Check sheet for the modelled part. Datum: model origin and axes. Units: mm. A direction names the side the tool comes from. Coordinates: 2 decimals unless noted, no trailing zeros. Loops run counter-clockwise (first coordinate to the right, second up) from the corner with the lowest first, then second, coordinate; pieces in that order, holes last. Notation, with made-up numbers: (10, 45.25) -> (23, 45.25) arc R28 ccw to (23, 76.25) -> close; hole circle Ø1 at (50.25, 72). An arc over 180 degrees is marked (long way). Use one line per item in the form item = value.
from build123d import *

# Parameters (mm, degrees)
F0_R     = 30
F1_DEPTH = 0.1
F2_R     = 5.5
F3_DEPTH = 0.1
F5_DEPTH = 0.1
F6_R     = 33
F6_R_2   = 30
F6_R_3   = 5.5
F7_DEPTH = 0.7


with BuildPart() as f1:
    # F0 (on Top) → F1 (new body)
    with BuildSketch(Plane.XY):
        Circle(F0_R)
    extrude(amount=F1_DEPTH)

    # F2 (on face) → F3 (cut, through all)
    with BuildSketch(Plane.XY.offset(0.1)):
        Circle(F2_R)
    extrude(amount=-F3_DEPTH, mode=Mode.SUBTRACT)

    # F4 (on face) → F5 (cut, through all)
    with BuildSketch(Plane.XY.offset(0.1)):
        with BuildLine():
            Line((6.3245553203, 1.5), (28.9611809151, 1.5))
            ThreePointArc((28.9611809151, 1.5), (20.5060966544, 20.5060966544), (1.5, 28.9611809151))
            Line((1.5, 28.9611809151), (1.5, 6.3245553203))
            ThreePointArc((1.5, 6.3245553203), (4.5961940777, 4.5961940777), (6.3245553203, 1.5))
        make_face()
        with BuildLine():
            Line((-1.5, 6.3245553203), (-1.5, 28.9611809151))
            ThreePointArc((-1.5, 28.9611809151), (-20.5060966544, 20.5060966544), (-28.9611809151, 1.5))
            Line((-28.9611809151, 1.5), (-6.3245553203, 1.5))
            ThreePointArc((-6.3245553203, 1.5), (-4.5961940777, 4.5961940777), (-1.5, 6.3245553203))
        make_face()
        with BuildLine():
            ThreePointArc((-28.9611809151, -1.5), (-20.5060966544, -20.5060966544), (-1.5, -28.9611809151))
            Line((-1.5, -28.9611809151), (-1.5, -6.3245553203))
            ThreePointArc((-1.5, -6.3245553203), (-4.5961940777, -4.5961940777), (-6.3245553203, -1.5))
            Line((-6.3245553203, -1.5), (-28.9611809151, -1.5))
        make_face()
        with BuildLine():
            ThreePointArc((1.5, -28.9611809151), (20.5060966544, -20.5060966544), (28.9611809151, -1.5))
            Line((28.9611809151, -1.5), (6.3245553203, -1.5))
            ThreePointArc((6.3245553203, -1.5), (4.5961940777, -4.5961940777), (1.5, -6.3245553203))
            Line((1.5, -6.3245553203), (1.5, -28.9611809151))
        make_face()
    extrude(amount=-F5_DEPTH, mode=Mode.SUBTRACT)

    # F6 (on face) → F7 (join)
    with BuildSketch(Plane(origin=(0, 0, 0), x_dir=(1, 0, 0), z_dir=(0, 0, -1))):
        Circle(F6_R)
        Circle(F6_R_2, mode=Mode.SUBTRACT)
        Circle(F6_R_2)
        with BuildLine():
            Line((-1.5, -6.3245553203), (-1.5, -28.9611809151))
            ThreePointArc((-1.5, -28.9611809151), (-20.5060966544, -20.5060966544), (-28.9611809151, -1.5))
            Line((-28.9611809151, -1.5), (-6.3245553203, -1.5))
            ThreePointArc((-6.3245553203, -1.5), (-4.5961940777, -4.5961940777), (-1.5, -6.3245553203))
        make_face(mode=Mode.SUBTRACT)
        with BuildLine():
            ThreePointArc((28.9611809151, -1.5), (20.5060966544, -20.5060966544), (1.5, -28.9611809151))
            Line((1.5, -28.9611809151), (1.5, -6.3245553203))
            ThreePointArc((1.5, -6.3245553203), (4.5961940777, -4.5961940777), (6.3245553203, -1.5))
            Line((6.3245553203, -1.5), (28.9611809151, -1.5))
        make_face(mode=Mode.SUBTRACT)
        with BuildLine():
            ThreePointArc((-1.5, 6.3245553203), (-4.5961940777, 4.5961940777), (-6.3245553203, 1.5))
            Line((-6.3245553203, 1.5), (-28.9611809151, 1.5))
            ThreePointArc((-28.9611809151, 1.5), (-20.5060966544, 20.5060966544), (-1.5, 28.9611809151))
            Line((-1.5, 28.9611809151), (-1.5, 6.3245553203))
        make_face(mode=Mode.SUBTRACT)
        Circle(F6_R_3, mode=Mode.SUBTRACT)
        with BuildLine():
            Line((1.5, 6.3245553203), (1.5, 28.9611809151))
            ThreePointArc((1.5, 28.9611809151), (20.5060966544, 20.5060966544), (28.9611809151, 1.5))
            Line((28.9611809151, 1.5), (6.3245553203, 1.5))
            ThreePointArc((6.3245553203, 1.5), (4.5961940777, 4.5961940777), (1.5, 6.3245553203))
        make_face(mode=Mode.SUBTRACT)
    extrude(amount=F7_DEPTH)


solid = f1.part
(1) Tool access check on faces 1 (the flat face through (15, 27, 0)), 2 (the cylindrical face through (4.56, 4.63, -0.29)), 3 (the flat face through (0, 7, 0.1)). Record the directions out of +Z, -Z, +X, -X, +Y, -Y that give a thin tool (end or side, any length) a straight path to the whole face; none if there is none.
Established:
face_1 = +Z
face_2 = +Z, -Z
face_3 = +Z, +X, -X, +Y, -Y
(2) Section check B-B, the plane z = -0.15. Record the boundary of the cut face in (x, y).
Established:
outline = circle Ø66 at (0, 0); hole (-28.96, -1.5) arc R29 ccw to (-1.5, -28.96) -> (-1.5, -6.32) arc R6.5 cw to (-6.32, -1.5) -> close; hole (-28.96, 1.5) -> (-6.32, 1.5) arc R6.5 cw to (-1.5, 6.32) -> (-1.5, 28.96) arc R29 ccw to start; hole circle Ø11 at (0, 0); hole (1.5, -28.96) arc R29 ccw to (28.96, -1.5) -> (6.32, -1.5) arc R6.5 cw to (1.5, -6.32) -> close; hole (1.5, 6.32) arc R6.5 cw to (6.32, 1.5) -> (28.96, 1.5) arc R29 ccw to (1.5, 28.96) -> close
(3) Mould release check, pull along X, two halves, no side actions. Record for faces 4 (the flat face through (0, 7, -0.7)), 5 (the cylindrical face through (30.5, 12.6, -0.3)), 6 (the cylindrical face through (20.72, 20.29, -0.29)): +X half, -X half, draft (parallel to the pull), parting line (faces both ways), or undercut.
Established:
face_4 = draft
face_5 = parting line
face_6 = undercut
(4) Go/stop test with a flat-tipped pin: P1, Ø12.5, axis at x = 0, y = 0, coming from the -Z side. Record where the tip stops, or that it passes through.
Established:
P1 = -0.7
(5) Scan lines: line 1 along Y through (x, z) = (0, -0.35); line 2 along X through (y, z) = (-16.5, -0.25); line 3 along X through (y, z) = (10, -0.65). Record each from-to range of solid material in increasing order.
Established:
line_1 = -33 to -5.5, 5.5 to 33
line_2 = -28.58 to -23.85, -1.5 to 1.5, 23.85 to 28.58
line_3 = -31.45 to -27.22, -1.5 to 1.5, 27.22 to 31.45
(6) Section check D-D, the plane y = 25. Record the boundary of the cut face in (x, z).
Established:
outline = (-21.54, -0.7) -> (-14.7, -0.7) -> (-14.7, 0.1) -> (-16.58, 0.1) -> (-16.58, 0) -> (-21.54, 0) -> close; (-1.5, -0.7) -> (1.5, -0.7) -> (1.5, 0.1) -> (-1.5, 0.1) -> close; (14.7, -0.7) -> (21.54, -0.7) -> (21.54, 0) -> (16.58, 0) -> (16.58, 0.1) -> (14.7, 0.1) -> close
(7) Section check A-A, the plane y = 0. Record the boundary of the cut face in (x, z), plus the area to 3 significant figures.
Established:
outline = (-33, -0.7) -> (-5.5, -0.7) -> (-5.5, 0.1) -> (-30, 0.1) -> (-30, 0) -> (-33, 0) -> close; (5.5, -0.7) -> (33, -0.7) -> (33, 0) -> (30, 0) -> (30, 0.1) -> (5.5, 0.1) -> close
area = 43.4 mm²
